Autodesk Inventor part; units mm, degrees
ref_plane "YZ Plane" through (0, 0, 0) normal (1, 0, 0) x (0, 1, 0)
ref_plane "XZ Plane" through (0, 0, 0) normal (0, 1, 0) x (-1, 0, 0)
ref_plane "XY Plane" through (0, 0, 0) normal (0, 0, 1) x (1, 0, 0)
sketch "スケッチ1" plane through (0, 0, 0) normal (1, 0, 0) x (0, 1, 0)
  line L0 (-30, 0) -> (-30, 21)
  line L1 (-30, 21) -> (0, 21)
  line L2 (0, 21) -> (0, 0)
  line L3 (-30, 0) -> (-30, -21)
  line L4 (-30, -21) -> (0, -21)
  line L5 (0, -21) -> (0, 0)
  arc A0 (0, -21) -> (0, 21) centre (0, 0) ccw
  dimension "d0" = 30
  dimension "d1" = 21
extrude "押し出し1" add sketch "スケッチ1" along normal mid plane 60
sketch "スケッチ2" plane through (30, 0, 0) normal (1, 0, 0) x (0, 0, -1)
  arc A0 (-12.5, 0) -> (12.5, 0) centre (0, 0) ccw
  arc A1 (21, 0) -> (-21, 0) centre (0, 0) ccw
  line L0 (-21, 0) -> (-12.5, 0)
  line L1 (12.5, 0) -> (21, 0)
  dimension "d4" = 25
extrude "押し出し2" cut sketch "スケッチ2" against normal blind 30
sketch "スケッチ3" plane through (0, 0, 0) normal (0, 1, 0) x (-1, 0, 0)
  line L0 (0, 0) -> (-4.5, 0)
  line L1 (-4.5, 0) -> (-4.5, 20)
  line L2 (-4.5, 20) -> (0, 20)
  line L3 (0, 20) -> (0, 0)
  line L4 (42, 0) -> (-42, 0)
  dimension "d7" = 4.5
  dimension "d8" = 20
revolve "回転1" cut sketch "スケッチ3" angle 360 about axis through (-10, 0, 0) along (1, 0, 0)
sketch "スケッチ4" plane through (0, 0, 0) normal (1, 0, 0) x (0, 0, -1)
  circle A0 centre (0, 0) radius 12
  dimension "d15" = 24
extrude "押し出し3" cut sketch "スケッチ4" against normal blind 20
sketch "スケッチ6" plane through (0, 0, 0) normal (0, 1, 0) x (-1, 0, 0)
  line L0 (20, -12) -> (20, 12)
  line L1 (20, 0) -> (24, 0)
  line L2 (24, 0) -> (24, 12.75)
  line L3 (24, 12.75) -> (20, 12.75)
  line L4 (20, 12.75) -> (20, 0)
  line L5 (42, 0) -> (-42, 0)
  point P0 (0, 0)
  dimension "d16" = 4
  dimension "d17" = 12.75
revolve "回転3" cut sketch "スケッチ6" angle 360 about axis through (-10, 0, 0) along (1, 0, 0)
sketch "スケッチ7" plane through (-30, 0, 0) normal (-1, 0, 0) x (0, 0, 1)
  circle A0 centre (0, 0) radius 11
  dimension "d19" = 22
extrude "押し出し4" cut sketch "スケッチ7" against normal through all
sketch "スケッチ8" plane through (0, 0, 0) normal (0, 1, 0) x (-1, 0, 0)
  line L0 (20, 12.75) -> (24, 12.75)
  line L1 (24, 0) -> (24, 12.75)
  line L2 (24, 12.75) -> (20, 12.75)
  line L3 (20, 12.75) -> (20, 0)
  line L4 (20, -12.75) -> (24, -12.75)
  line L5 (24, 0) -> (24, -12.75)
  line L6 (20, -12.75) -> (20, 0)
  point P0 (0, 0)
extrude "押し出し5" cut sketch "スケッチ8" along normal through all
sketch "スケッチ9" plane through (0, 0, 0) normal (0, 1, 0) x (-1, 0, 0)
  line L0 (24, 0) -> (24, -5.5)
  line L1 (24, -5.5) -> (20, -5.5)
  line L2 (20, -5.5) -> (20, 0)
  line L3 (24, 0) -> (24, 5.5)
  line L4 (24, 5.5) -> (20, 5.5)
  line L5 (20, 5.5) -> (20, 0)
  point P0 (0, 0)
  dimension "d24" = 4
  dimension "d25" = 5.5
extrude "押し出し6" cut sketch "スケッチ9" against normal through all
sketch "スケッチ10" plane through (-30, -30, -21) normal (0, -1, 0) x (1, 0, 0)
  line L0 (30, 21) -> (20, 21) construction
  circle A0 centre (20, 21) radius 4
  dimension "d28" = 10
  dimension "d29" = 8
extrude "押し出し7" cut sketch "スケッチ10" against normal blind 10
properties part number "raman-colimeter-holder" material "ABS プラスチック"
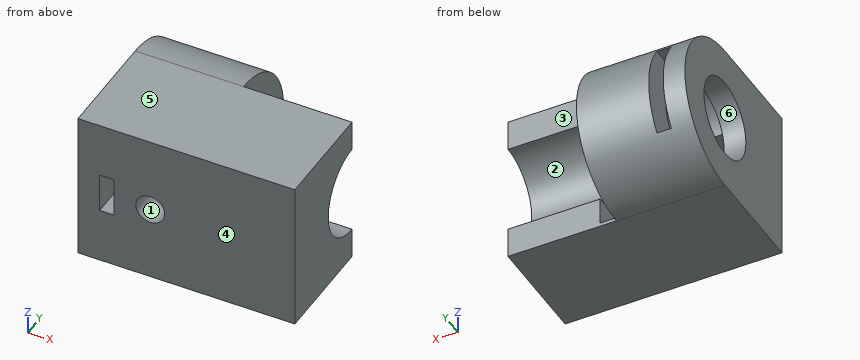
Work out the finished part from the listing and answer in its coordinate system (mm). Face numbers are marked on the shaded views. A direction names the side the tool comes from. Round coordinates to 2 decimals unless told otherwise and drop trailing zeros. Write each loop counter-clockwise with the first axis right and the second up, starting at its lowest first coordinate (ties: lowest second). Pieces come first, ordered by that corner, then holes.
1) A cutting plane is placed at A-A on z = 0. Determine the outline of the cut face in (x, y), and give its area (3 significant figures).
2) Consider probe 1 along X at (y, z) = (-15, 4.5); probe 2 along Y at (x, z) = (-28.7, 0); probe 3 along X at (y, z) = (7.5, 12). Determine where each line is inside the solid, lowest interval first.
3) A cutting plane is placed at B-B on y = -26. Determine the outline of the cut face in (x, z), and give its area (3 significant figures).
4) A cutting plane is placed at D-D on z = -10. Determine the outline of the cut face in (x, y), and give its area (3 significant figures).
5) A cutting plane is placed at C-C on x = -10. Determine the outline of the cut face in (y, z).
6) Determine the mould class of the marked faces 4, 5 and 6 for opening direction Y: pulls with the +Y half, pulls with the -Y half, needs draft (parallel to the pull), parting line crosses it, or undercut.
7) Which of the six approach directions +Z, -Z, +X, -X, +Y, -Y give full straight-line access (tool end or side, diameter ignored) to the marked faces 1, 2 and 3?
8) Flat-ended cylindrical pins translate along their axes: P1, Ø3, axis at x = -23, y = 8.5, coming from the +Z side; P2, Ø1.5, axis at x = 23, z = -6.5, coming from the +Y side; P3, Ø7, axis at x = 13, z = -17.5, coming from the +Y side. Find the tip coordinate at first contact, or state that the pin passes through.
Entries:
1. outline: (-30, -30) - (-24, -30) - (-24, -11) - (-30, -11) - close; (-30, 11) - (-24, 11) - (-24, 21) - (-30, 21) - close; (-20, -30) - (-14, -30) - (-14, -20) - (-6, -20) - (-6, -30) - (30, -30) - (30, -12.5) - (4.5, -12.5) - (4.5, -20) - (0, -20) - (0, -12) - (-20, -12) - close; (-20, 12) - (0, 12) - (0, 21) - (-20, 21) - close
1. area: 1,130 mm2
2. probe 1: x = -30 to -24, -20 to 0, 4.5 to 30
2. probe 2: y = -30 to -11, 11 to 21
2. probe 3: x = -30 to -24, -20 to 0
3. outline: (-30, -21) - (30, -21) - (30, 21) - (-30, 21) - close; hole (-24, -5.5) - (-20, -5.5) - (-20, 5.5) - (-24, 5.5) - close; hole circle Ø8 at (-10, 0)
3. area: 2,430 mm2
4. outline: (-30, -30) - (30, -30) - (30, -7.5) - (4.5, -7.5) - (4.5, -17.32) - (0, -17.32) - (0, -6.63) - (-20, -6.63) - (-20, -7.91) - (-24, -7.91) - (-24, -4.58) - (-30, -4.58) - close; (-30, 4.58) - (-24, 4.58) - (-24, 18.47) - (-30, 18.47) - close; (-20, 6.63) - (0, 6.63) - (0, 18.47) - (-20, 18.47) - close
4. area: 1,660 mm2
5. outline: (-30, -21) - (0, -21) arc R21 ccw to (0, 21) - (-30, 21) - (-30, 4) - (-20, 4) - (-20, -4) - (-30, -4) - close; hole circle Ø24 at (0, 0)
6. face 4: pulls with the -Y half
6. face 5: needs draft
6. face 6: undercut
7. face 1: -Y
7. face 2: +X, +Y
7. face 3: +Z, -Z, +X, +Y
8. P1: stops at z = 19.8
8. P2: stops at y = -10.18
8. P3: stops at y = 0
